The figure shows three views and two pictorial views of one solid part (mm, origin at its lowest corner). Answer the questions. A direction names the side the tool comes from. Give positions to 0.01 mm unless a question says otherwise; leave off trailing zeros. Order: outer loops, then holes, each group sorted by start corner. A loop starts at its lowest first (then second) coordinate and runs counter-clockwise, first axis right, second up. Notation, with made-up numbers: (16.25, -15.75) - (59.25, -15.75) arc R34 cw to (59.25, 20.25) - close; hole circle Ø10 at (-15.5, -5.5). An arc over 180 degrees is marked (long way). Write item = value, one per line.
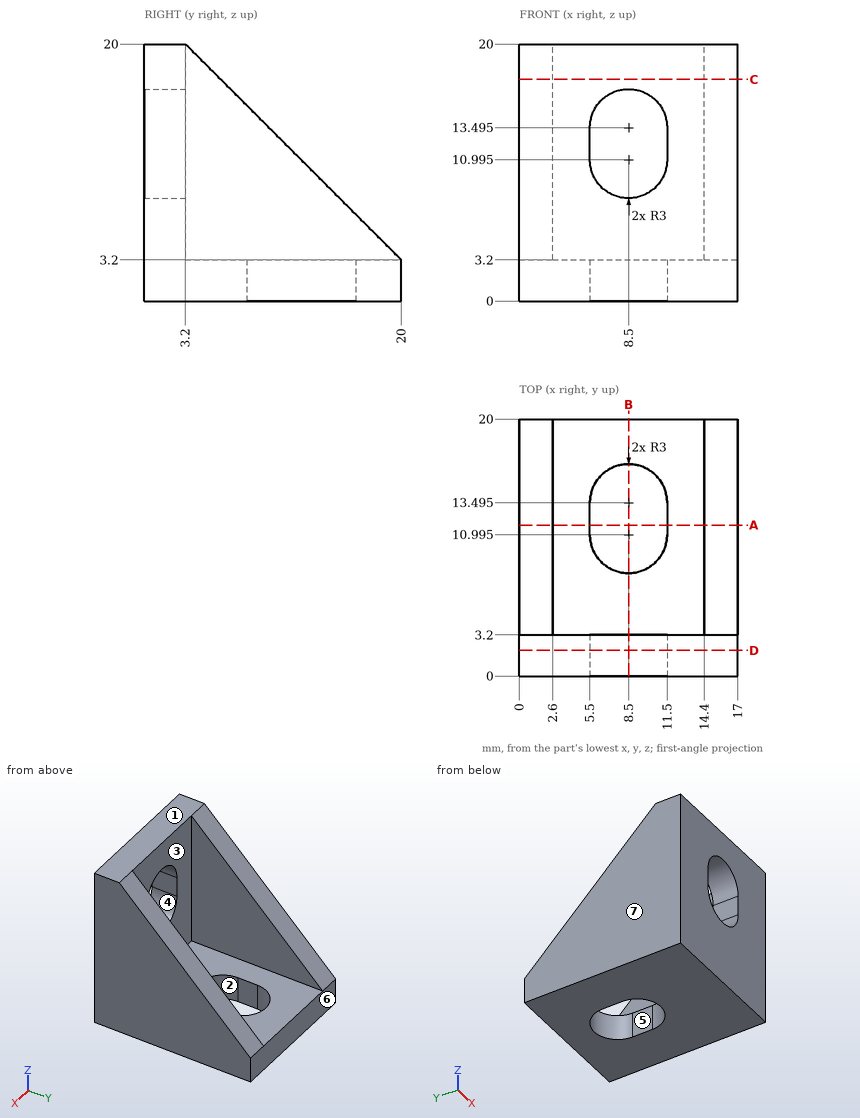
1. Section C-C (z = 17.25) is taken. Determine the outline of the cut face in (x, y).
Recorded:
outline = (0, 0) - (17, 0) - (17, 5.95) - (14.4, 5.95) - (14.4, 3.2) - (2.6, 3.2) - (2.6, 5.95) - (0, 5.95) - close
2. Section B-B (x = 8.5) is taken. Determine the outline of the cut face in (y, z) (3 decimals), and give its area (3 significant figures).
Recorded:
outline = (0, 0) - (7.995, 0) - (7.995, 3.2) - (3.2, 3.2) - (3.2, 7.995) - (0, 7.995) - close; (0, 16.495) - (3.2, 16.495) - (3.2, 20) - (0, 20) - close; (16.495, 0) - (20, 0) - (20, 3.2) - (16.495, 3.2) - close
area = 63.4 mm^2
3. Straight lines are drawn through the part: L1, parallel to X at y = 10.5, z = 5; L2, parallel to Z at x = 2.75, y = 17.25. For each, find the intervals that lie inside material, in ascending order. Write a range as [from, to].
Recorded:
L1 = [0, 2.6], [14.4, 17]
L2 = [0, 3.2]
4. Section D-D (y = 2) is taken. Determine the outline of the cut face in (x, z) (3 decimals).
Recorded:
outline = (0, 0) - (17, 0) - (17, 20) - (0, 20) - close; hole (5.5, 10.995) arc R3 ccw to (11.5, 10.995) - (11.5, 13.495) arc R3 ccw to (5.5, 13.495) - close
5. Section A-A (y = 11.75) is taken. Determine the outline of the cut face in (x, z).
Recorded:
outline = (0, 0) - (5.5, 0) - (5.5, 3.2) - (2.6, 3.2) - (2.6, 11.45) - (0, 11.45) - close; (11.5, 0) - (17, 0) - (17, 11.45) - (14.4, 11.45) - (14.4, 3.2) - (11.5, 3.2) - close
6. A flat-ended cylindrical pin translates along its axis: pin 1 (1 mm diameter, centred on x = 5, z = 12, fed in from +Y). Find the tip coordinate at first contact, or state that the pin passes through.
Recorded:
pin_1 = 3.2
7. For the marked faces 1, 2, 3 and 4, determine the directions among +Z, -Z, +X, -X, +Y, -Y from which every point of the face is accessible in a straight line to the end or side of a thin tool.
Recorded:
face_1 = +Z, +X, -X, +Y, -Y
face_2 = +Z, -Z
face_3 = +Z, +Y
face_4 = +Y, -Y
8. Determine the mould class of the marked faces 5, 6 and 7 for opening direction X: +X half, -X half, draft (parallel to the pull), parting line (faces both ways), or undercut.
Recorded:
face_5 = undercut
face_6 = draft
face_7 = -X half
